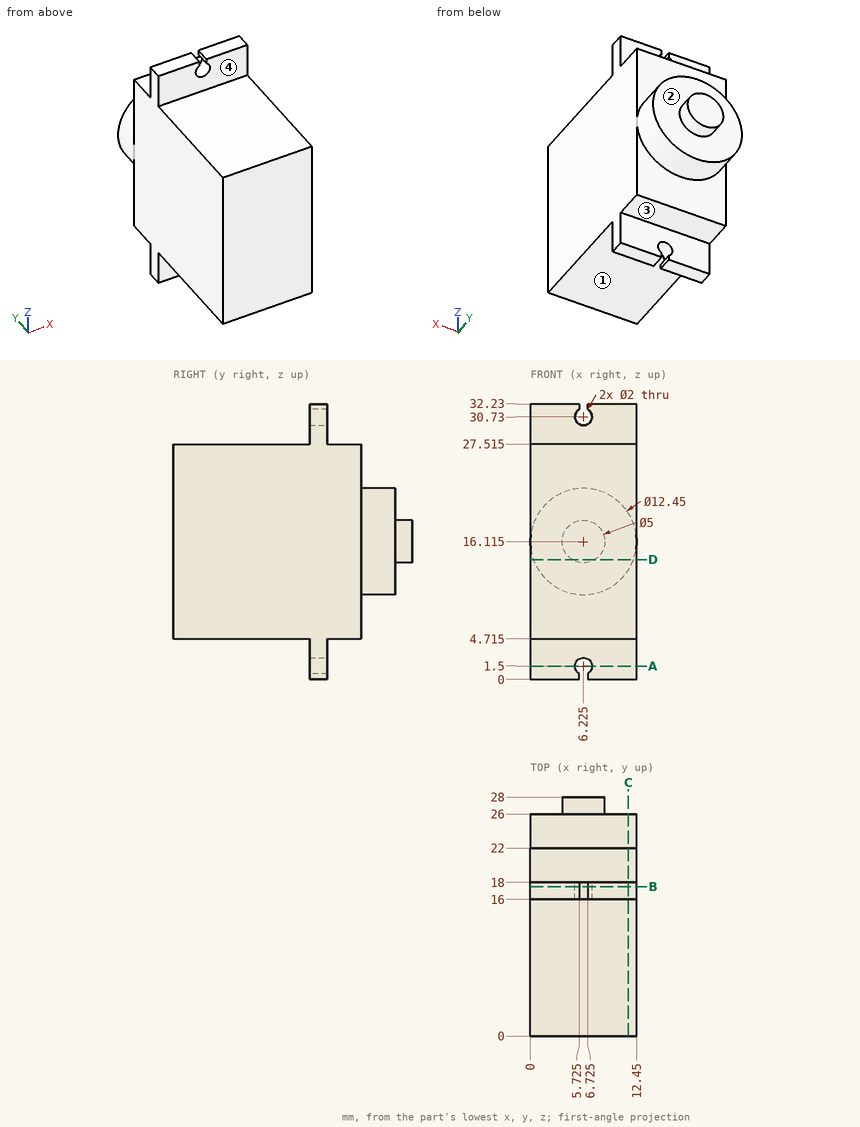
Input: dimensioned drawing with shaded views. Units: mm. Origin: part minimum x, y, z. A direction names the side the tool comes from. Coordinates: 2 decimals unless noted, no trailing zeros. Loops run counter-clockwise (first coordinate to the right, second up) from the corner with the lowest first, then second, coordinate; pieces in that order, holes last. Notation, with made-up numbers: M -35.5,60.25 L -26.5,60.25 A27 ccw -26.5,95.25 Z; hole C -37.75,44 d4. An arc over 180 degrees is marked long. One line per item, written item: value. Start each with the question number.
1) Cut plane C-C (x = 11.5). Return loops of the section in (y, z) (3 decimals).
2) Material intervals for L1, parallel to X at y = 17.5, z = 30.73 (3 decimals); L2, parallel to Z at x = 1.25, y = 13.75 (3 decimals); L3, parallel to Y at x = 12.25, z = 7, sorted ascending. Write a range as from..to.
3) Reachability of the marked faces 1, 2, 3 and 4 from +Z, -Z, +X, -X, +Y, -Y: full face, straight path, thin tool, end or side. Return the list, or none.
4) Cut plane B-B (y = 17.5). Return loops of the section in (x, z) (3 decimals).
5) Cut plane A-A (z = 1.5). Return loops of the section in (x, y) (3 decimals).
6) Cut plane D-D (z = 14). Return loops of the section in (x, y), then the cut area to 3 significant figures.
7) Pin query (flat end, axial travel): P1, Ø5, axis at x = 3.5, z = 30.5, coming from the +Y side; P2, Ø3, axis at x = 9, y = 20, coming from the +Z side (3 decimals); P3, Ø4, axis at y = 25, z = 7, coming from the -X side; P4, Ø1.2, axis at x = 3, y = 20.5, coming from the -Z side (3 decimals). Return the tip coordinate at first contact, or that it passes through.
Evaluation:
1. outline: M 0,4.715 L 16,4.715 L 16,0 L 18,0 L 18,4.715 L 22,4.715 L 22,12.81 L 26,12.81 L 26,19.42 L 22,19.42 L 22,27.515 L 18,27.515 L 18,32.23 L 16,32.23 L 16,27.515 L 0,27.515 Z
2. L1: 0..5.225, 7.225..12.45
2. L2: 4.715..27.515
2. L3: 0..22
3. face 1: -Z, +X, -X, -Y
3. face 2: +Y
3. face 3: -Z, +X, -X, +Y
3. face 4: +Z, +X, -X, -Y
4. outline: M 0,0 L 5.725,0 L 5.725,0.634 A1 cw long 6.725,0.634 L 6.725,0 L 12.45,0 L 12.45,32.23 L 6.725,32.23 L 6.725,31.596 A1 cw long 5.725,31.596 L 5.725,32.23 L 0,32.23 Z
5. outline: M 0,16 L 5.225,16 L 5.225,18 L 0,18 Z; M 7.225,16 L 12.45,16 L 12.45,18 L 7.225,18 Z
6. outline: M 0,0 L 12.45,0 L 12.45,22 L 12.08,22 L 12.08,26 L 7.56,26 L 7.56,28 L 4.89,28 L 4.89,26 L 0.37,26 L 0.37,22 L 0,22 Z
6. area: 326 mm^2
7. P1: y = 18
7. P2: z = 27.515
7. P3: through
7. P4: z = 4.715
